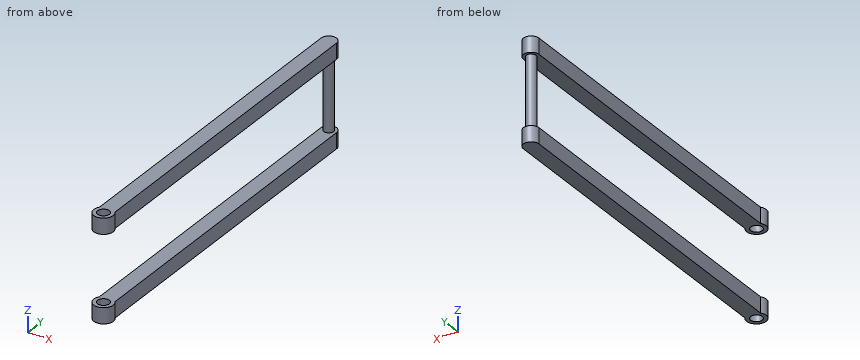
```python
from build123d import *

# Parameters (mm, degrees)
SKETCH1_R                = 1.25
SKETCH1_R_2              = 1.5
BOSS_EXTRUDE1_DEPTH      = 2
BOSS_EXTRUDE1_DEPTH_BACK = 2
SKETCH1_4_R              = 1.25
BOSS_EXTRUDE2_DEPTH      = 20


with BuildPart() as part:
    # Sketch1 → Boss-Extrude1 (new, two sides)
    with BuildSketch(Plane.XY) as boss_extrude1_sk:
        with BuildLine():
            ThreePointArc((2, 1.5), (0, -2.5), (-2, 1.5))
            Line((-2, 1.5), (-2, 90))
            ThreePointArc((-2, 90), (0, 92), (2, 90))
            Line((2, 90), (2, 1.5))
        make_face()
        with Locations((0, 90)):
            Circle(SKETCH1_R, mode=Mode.SUBTRACT)
        Circle(SKETCH1_R_2, mode=Mode.SUBTRACT)
        with Locations((0, 90)):
            Circle(SKETCH1_R)
    extrude(amount=BOSS_EXTRUDE1_DEPTH)
    extrude(boss_extrude1_sk.sketch, amount=-BOSS_EXTRUDE1_DEPTH_BACK)


with BuildPart() as body_2:
    # Mirror2: mirrored copy
    add(part.part.mirror(Plane.XY.offset(11)))


with BuildPart() as part_1:
    add(part.part)

    add(body_2.part)  # Boss-Extrude2 merges body 2
    # Sketch1<4> → Boss-Extrude2 (add)
    with BuildSketch(Plane.XY):
        with Locations(Location((0, 90, 0), (0, 0, 180))):
            Circle(SKETCH1_4_R)
    extrude(amount=BOSS_EXTRUDE2_DEPTH)


solid = part_1.part
```
Here's how the part is built. I have some questions about the finished solid (model axes, mm). Give positions to 0.01 mm unless a question says otherwise; leave off trailing zeros. Order: outer loops, then holes, each group sorted by start corner. A loop starts at its lowest first (then second) coordinate and runs counter-clockwise, first axis right, second up. Notation, with made-up numbers: M -3.75,-12 L 6.25,-12 A32 ccw 6.25,24 Z; hole C 64.25,-28 d11. An arc over 180 degrees is marked long. Use a Markdown table: item, result. Add a question column.
1. Suppose I cut it at D-D (z = 11.5). List the corners of the cut face in (x, y) for me.
2. Suppose I cut it at C-C (y = 0). List the corners of the cut face in (x, z) for me, and give its area (3 significant figures).
3. Suppose I cut it at B-B (y = 12). List the corners of the cut face in (x, z) for me.
4. For pin 1 Ø4 at (y, z) = (65.5, 21) entering from +X; pin 2 Ø1.2 at (y, z) = (35.5, 1) entering from -X; pin 3 Ø1.5 at (x, z) = (1.5, 3.5) entering from -Y, each with a flat end and sliding along its axis, tell me the tip position at first contact or that it passes through.
5. Suppose I cut it at A-A (x = 0). List the corners of the cut face in (y, z) for me.
6. I need wall thicknesses on probe 1 along Z at (x, y) = (-1.2, 2); probe 2 along X at (y, z) = (69, 22.25); probe 3 along Y at (x, z) = (1.35, -0.5). Which ranges of each line are inside material? Lowest first, please. Write a range as from..to.
Results list:
| question | item | result |
|---|---|---|
| 1 | outline | C 0,90 d2.5 |
| 2 | outline | M -2.5,-2 L -1.5,-2 L -1.5,2 L -2.5,2 Z; M -2.5,20 L -1.5,20 L -1.5,24 L -2.5,24 Z; M 1.5,-2 L 2.5,-2 L 2.5,2 L 1.5,2 Z; M 1.5,20 L 2.5,20 L 2.5,24 L 1.5,24 Z |
| 2 | area | 16.0 mm² |
| 3 | outline | M -2,-2 L 2,-2 L 2,2 L -2,2 Z; M -2,20 L 2,20 L 2,24 L -2,24 Z |
| 4 | pin 1 | stops at x = 2 |
| 4 | pin 2 | stops at x = -2 |
| 4 | pin 3 | stops at y = 89 |
| 5 | outline | M -2.5,-2 L -1.5,-2 L -1.5,2 L -2.5,2 Z; M -2.5,20 L -1.5,20 L -1.5,24 L -2.5,24 Z; M 1.5,-2 L 92,-2 L 92,2 L 91.25,2 L 91.25,20 L 92,20 L 92,24 L 1.5,24 L 1.5,20 L 88.75,20 L 88.75,2 L 1.5,2 Z |
| 6 | probe 1 | z = -2..2, 20..24 |
| 6 | probe 2 | x = -2..2 |
| 6 | probe 3 | y = -2.1..-0.65, 0.65..91.48 |
